Autodesk Inventor part; units mm, degrees
ref_plane "YZ Plane" through (0, 0, 0) normal (1, 0, 0) x (0, 1, 0)
ref_plane "XZ Plane" through (0, 0, 0) normal (0, 1, 0) x (-1, 0, 0)
ref_plane "XY Plane" through (0, 0, 0) normal (0, 0, 1) x (1, 0, 0)
sketch "Sketch1" plane through (0, 0, 0) normal (0, 0, 1) x (1, 0, 0)
  circle A0 centre (0, 0) radius 11
  circle A1 centre (0, 0) radius 4
  dimension "d0" = 22
  dimension "d1" = 8
extrude "Extrusion1" add sketch "Sketch1" along normal mid plane 7
sketch "Sketch2" plane through (0, 0, 3.5) normal (0, 0, 1) x (1, 0, 0)
  circle A0 centre (0, 0) radius 10
  circle A1 centre (0, 0) radius 5
  circle A2 centre (0, 0) radius 11
  circle A3 centre (0, 0) radius 4
  dimension "d4" = 1
  dimension "d5" = 1
extrude "Extrusion2" cut sketch "Sketch2" against normal blind 0.5 contours A0
mirror "Mirror1" about plane through (0, 0, 0) normal (0, 0, 1) of "Extrusion2"
chamfer "Chamfer1" distance 0.15 angle 45 8 edges at (-11, 0, 3.5) (-11, 0, -3.5) (-10, 0, 3.5) (-5, 0, 3.5) (-4, 0, 3.5) (-10, 0, -3.5) (-5, 0, -3.5) (-4, 0, -3.5)
properties part number "SS608-2RS"
CAD build for the part. Positions are in the model's coordinates, mm. A direction names the side the tool comes from. Coordinates: 2 decimals unless noted, no trailing zeros. Write each loop counter-clockwise with the first axis right and the second up, starting at its lowest first coordinate (ties: lowest second). Pieces come first, ordered by that corner, then holes. Notation, with made-up numbers: M -24,10.25 L -17,10.25 A10 ccw -17,27.25 Z; hole C 50,22.25 d9. An arc over 180 degrees is marked long. Return JSON: item names as keys, results as strings.
Item 1: Drop flat-ended pins along their axis: pin 1 Ø1 at (x, y) = (-0.5, -8.5) entering from +Z; pin 2 Ø1 at (y, z) = (-6, -2) entering from -X; pin 3 Ø2 at (x, y) = (1.5, 8.5) entering from -Z. Give the stop position or say it passes through.
Findings below:
{"pin 1": "stops at z = 3", "pin 2": "stops at x = -9.53", "pin 3": "stops at z = -3"}
Item 2: Two-plate mould, pull along Y, no slides. Class faces 1 (the flat face through (2, 5, 3)), 2 (the cylindrical face through (-2.38, 10.74, -0.05)), 3 (the flat face through (9.6, -4, -3.5)): +Y half, -Y half, draft (parallel to the pull), parting line (faces both ways), or undercut.
Findings below:
{"face 1": "undercut", "face 2": "parting line", "face 3": "draft"}
Item 3: Probe line 1 (Y direction, x = 0, z = -3.1); line 2 (Y direction, x = 0, z = -0.75); line 3 (Z direction, x = 0.5, y = 9). List the from-to ranges inside material, lowest first. Write a range as from..to.
Findings below:
{"line 1": "y = -11..-10, -5..-4, 4..5, 10..11", "line 2": "y = -11..-4, 4..11", "line 3": "z = -3..3"}
Item 4: Which spindle directions (+Z, -Z, +X, -X, +Y, -Y) get a long thin tool onto all of the face, cutting with end or side? Do faces 4 (the cylindrical face through (-1.08, -4.88, 3.18)), 5 (the cylindrical face through (-1.08, 4.88, -3.18)), 6 (the cylindrical face through (-0.867, -3.905, 0.047)). Say none if no direction does.
Findings below:
{"face 4": "+Z", "face 5": "-Z", "face 6": "+Z, -Z"}
Item 5: Slice it at A-A, the plane z = -1.25. Write the cut outline in (x, y), and give its area (3 significant figures).
Findings below:
{"outline": "C 0,0 d22; hole C 0,0 d8", "area": "330 mm2"}
